For this review, take the finished solid that the model builds, in its own axes (mm). Face numbers are marked on the shaded views. A direction names the side the tool comes from. Coordinates: 2 decimals unless noted, no trailing zeros. Loops run counter-clockwise (first coordinate to the right, second up) from the corner with the lowest first, then second, coordinate; pieces in that order, holes last. Notation, with made-up numbers: M 20,-22.5 L 76,-22.5 A18 ccw 76,-6.5 Z; hole C -14.5,-10.5 d8. An arc over 180 degrees is marked long. Use one line per item in the form item = value.
```python
from build123d import *

# Parameters (mm, degrees)
SKETCH_1_W          = 150
SKETCH_1_H          = 60
EXTRUDE_1_DEPTH     = 6
SKETCH_2_W          = 10
SKETCH_2_H          = 60
EXTRUDE_2_DEPTH     = 22
SKETCH_3_W          = 6.2
SKETCH_3_H          = 55.2
CUT_EXTRUDE_1_DEPTH = 4
SKETCH_4_R          = 17
CUT_EXTRUDE_2_DEPTH = 129.716743278
SKETCH_5_W          = 20
SKETCH_5_H          = 52
SKETCH_5_W_2        = 62
CUT_EXTRUDE_3_DEPTH = 84.719770664


with BuildPart() as part:
    # 草图1 → 凸台-拉伸1 (new body)
    with BuildSketch(Plane(origin=(0, 0, 0), x_dir=(1, 0, 0), z_dir=(0, 1, 0))):
        Rectangle(SKETCH_1_W, SKETCH_1_H)
    extrude(amount=EXTRUDE_1_DEPTH)

    # 草图2 → 凸台-拉伸2 (add)
    with BuildSketch(Plane(origin=(0, 6, 0), x_dir=(1, 0, 0), z_dir=(0, 1, 0))):
        with Locations((-42, 0)):
            Rectangle(SKETCH_2_W, SKETCH_2_H)
        with Locations((42, 0)):
            Rectangle(SKETCH_2_W, SKETCH_2_H)
    extrude(amount=EXTRUDE_2_DEPTH)

    # 草图3 → 切除-拉伸1 (cut)
    with BuildSketch(Plane(origin=(0, 28, 0), x_dir=(1, 0, 0), z_dir=(0, 1, 0))):
        with Locations((-42, 0)):
            Rectangle(SKETCH_3_W, SKETCH_3_H)
        with Locations((42, 0)):
            Rectangle(SKETCH_3_W, SKETCH_3_H)
    extrude(amount=-CUT_EXTRUDE_1_DEPTH, mode=Mode.SUBTRACT)

    # 草图4 → 切除-拉伸2 (cut, through all)
    with BuildSketch(Plane.ZY.offset(47)):
        with Locations((0, 28)):
            Circle(SKETCH_4_R)
    extrude(amount=-CUT_EXTRUDE_2_DEPTH, mode=Mode.SUBTRACT)

    # 草图5 → 切除-拉伸3 (cut, through all)
    with BuildSketch(Plane(origin=(0, 6, 0), x_dir=(1, 0, 0), z_dir=(0, 1, 0))):
        with Locations((-61, 0)):
            Rectangle(SKETCH_5_W, SKETCH_5_H)
        with Locations((61, 0)):
            Rectangle(SKETCH_5_W, SKETCH_5_H)
        Rectangle(SKETCH_5_W_2, SKETCH_5_H)
    extrude(amount=-CUT_EXTRUDE_3_DEPTH, mode=Mode.SUBTRACT)


solid = part.part
```
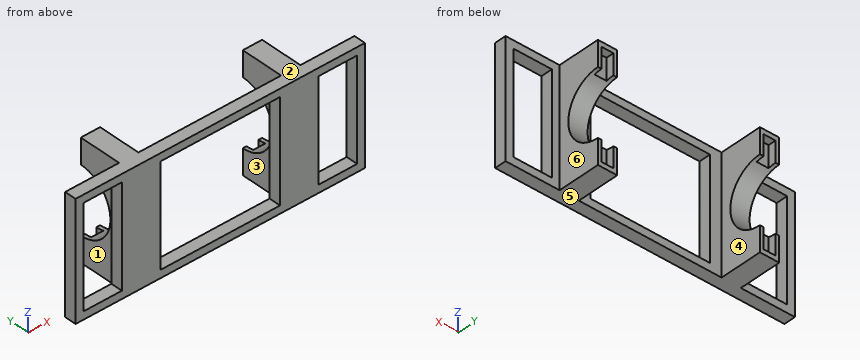
1. Wall thickness on line 1 along X through (y, z) = (10.5, -25); line 2 along Z through (x, y) = (18.5, 2.25); line 3 along X through (y, z) = (1.75, 17.5): over which ranges is each line inside the solid? List them lowest first. Write a range as from..to.
Computed values:
line_1 = -47..-37, 37..47
line_2 = -30..-26, 26..30
line_3 = -75..-71, -51..-31, 31..51, 71..75
2. For pin 1 Ø1.2 at (y, z) = (27, -25) entering from +X; pin 2 Ø1.9 at (x, z) = (41.5, -23.5) entering from +Y; pin 3 Ø1.2 at (y, z) = (26.5, 23.5) entering from -X, all flat-tipped, find the tip position at first contact; note any pin that passes through.
Computed values:
pin_1 = 47
pin_2 = 24
pin_3 = -47
3. Tool access review of the marked faces 1, 2 and 3: name each direction out of +Z, -Z, +X, -X, +Y, -Y from which nothing blocks a thin tool from reaching the whole face with its end or side.
Computed values:
face_1 = +Z, -Z, -X, +Y
face_2 = +Z, +X, -X, +Y, -Y
face_3 = +Z, -Z, +Y
4. Consider section D-D on z = 0. Write out the cut boundary in (x, y).
Computed values:
outline = M -75,0 L -71,0 L -71,6 L -75,6 Z; M -51,0 L -31,0 L -31,6 L -37,6 L -37,11 L -47,11 L -47,6 L -51,6 Z; M 31,0 L 51,0 L 51,6 L 47,6 L 47,11 L 37,11 L 37,6 L 31,6 Z; M 71,0 L 75,0 L 75,6 L 71,6 Z
5. Consider section B-B on y = 13. Write out the cut boundary in (x, z), plus the area to 3 significant figures.
Computed values:
outline = M -47,-30 L -37,-30 L -37,-8 L -47,-8 Z; M -47,8 L -37,8 L -37,30 L -47,30 Z; M 37,-30 L 47,-30 L 47,-8 L 37,-8 Z; M 37,8 L 47,8 L 47,30 L 37,30 Z
area = 880 mm2
6. Consider section C-C on x = -3. Write out the cut boundary in (y, z), plus the area to 3 significant figures.
Computed values:
outline = M 0,-30 L 6,-30 L 6,-26 L 0,-26 Z; M 0,26 L 6,26 L 6,30 L 0,30 Z
area = 48.0 mm2
7. Consider section A-A on z = -22.5. State how many separate pieces and enclosed holes the cut face has, plus the area to 3 significant figures.
Computed values:
separate_pieces = 4
enclosed_holes = 0
area = 678 mm2
8. Draft analysis for pull direction X (two halves, no side actions). For the marked faces 4, 5 and 6, state which applies: +X half, -X half, draft (parallel to the pull), parting line (faces both ways), or undercut.
Computed values:
face_4 = undercut
face_5 = draft
face_6 = +X half
